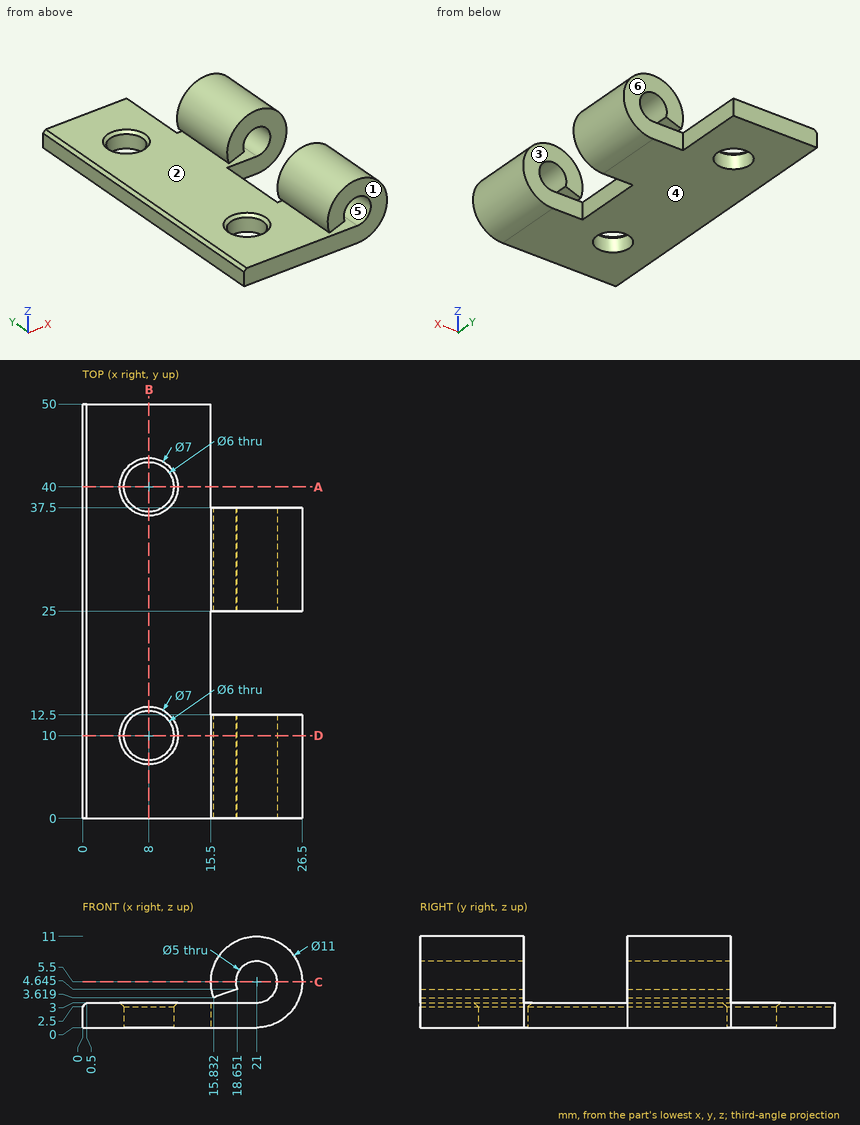
Here's the drawing with two shaded views (mm, measured from the low corner). I have some questions. A direction names the side the tool comes from. Give positions to 0.01 mm unless a question says otherwise; leave off trailing zeros. Loops run counter-clockwise (first coordinate to the right, second up) from the corner with the lowest first, then second, coordinate; pieces in that order, holes last. Notation, with made-up numbers: (28.25, 19) -> (69.25, 19) arc R19 ccw to (69.25, 28) -> close; hole circle Ø5 at (52, 75.5). An arc over 180 degrees is marked (long way). Use one line per item in the form item = value.
1) If we section it at C-C (z = 5.5): Please give me the cut outline in (x, y), plus the area to 3 significant figures.
Answers:
outline = (15.5, 0) -> (18.5, 0) -> (18.5, 12.5) -> (15.5, 12.5) -> close; (15.5, 25) -> (18.5, 25) -> (18.5, 37.5) -> (15.5, 37.5) -> close; (23.5, 0) -> (26.5, 0) -> (26.5, 12.5) -> (23.5, 12.5) -> close; (23.5, 25) -> (26.5, 25) -> (26.5, 37.5) -> (23.5, 37.5) -> close
area = 150 mm²
2) Will these pins go through, and if not, where does the flat tip stop? pin 1 (2 mm diameter, centred on x = 20, z = 6.5, fed in from +Y); pin 2 (1.5 mm diameter, centred on y = 13, z = 2, fed in from +X); pin 3 (0.9 mm diameter, centred on y = 21.5, z = 2, fed in from +X); pin 4 (1.5 mm diameter, centred on x = 15.5, z = 8, fed in from +Y).
Answers:
pin_1 = through
pin_2 = 25.65
pin_3 = 15.5
pin_4 = 37.5
3) I need wall thicknesses on line 1 along Y through (x, z) = (8, 1.1); line 2 along Y through (x, z) = (17, 8.25); line 3 along X through (y, z) = (33.5, 5.5). Which ranges of each line are inside material? Lowest first, please.
Answers:
line_1 = 0 to 7, 13 to 37, 43 to 50
line_2 = 0 to 12.5, 25 to 37.5
line_3 = 15.5 to 18.5, 23.5 to 26.5
4) We'd pull the mould along Z, two halves only. Please class the marked faces 4, 5 and 6: released by +Z, released by -Z, zero draft, split by the parting line, or undercut.
Answers:
face_4 = released by -Z
face_5 = undercut
face_6 = zero draft
5) If we section it at B-B (x = 8): Please give me the cut outline in (y, z).
Answers:
outline = (0, 0) -> (7, 0) -> (7, 2.5) -> (6.5, 3) -> (0, 3) -> close; (13, 0) -> (37, 0) -> (37, 2.5) -> (36.5, 3) -> (13.5, 3) -> (13, 2.5) -> close; (43, 0) -> (50, 0) -> (50, 3) -> (43.5, 3) -> (43, 2.5) -> close
6) If we section it at A-A (y = 40): Please give me the cut outline in (x, z), plus the area to 3 significant figures.
Answers:
outline = (0, 0) -> (5, 0) -> (5, 2.5) -> (4.5, 3) -> (0.5, 3) -> (0, 2.5) -> close; (11, 0) -> (15.5, 0) -> (15.5, 3) -> (11.5, 3) -> (11, 2.5) -> close
area = 28.1 mm²
7) For the marked faces 1, 2 and 3, which set-ups out of +Z, -Z, +X, -X, +Y, -Y let a thin tool reach every point of the face, with its end or its side?
Answers:
face_1 = +Z, -Z, +X, -X, -Y
face_2 = -X, +Y, -Y
face_3 = +Z, -Z, +X
8) If we section it at D-D (y = 10): Please give me the cut outline in (x, z) (1 decimal).
Answers:
outline = (0, 0) -> (5, 0) -> (5, 2.5) -> (4.5, 3) -> (0.5, 3) -> (0, 2.5) -> close; (11, 0) -> (21, 0) arc R5.5 ccw (long way) to (15.8, 3.6) -> (18.7, 4.6) arc R2.5 cw (long way) to (21, 3) -> (11.5, 3) -> (11, 2.5) -> close
